from build123d import *

# Parameters (mm, degrees)
SCHIZZO1_R                   = 47
SCHIZZO1_R_2                 = 35
ESTRUSIONE_ESTRUSIONE1_DEPTH = 4
SCHIZZO2_R                   = 2.25
TAGLIO_ESTRUSIONE1_DEPTH     = 4


with BuildPart() as part:
    # Schizzo1 → Estrusione-Estrusione1 (new body)
    with BuildSketch(Plane(origin=(0, 0, 0), x_dir=(1, 0, 0), z_dir=(0, 1, 0))):
        with Locations(Location((0, 0, 0), (0, 0, 270))):
            Circle(SCHIZZO1_R)
        with Locations(Location((0, 0, 0), (0, 0, 270))):
            Circle(SCHIZZO1_R_2, mode=Mode.SUBTRACT)
    extrude(amount=ESTRUSIONE_ESTRUSIONE1_DEPTH)

    # Schizzo2 → Taglio-Estrusione1 (cut)
    with BuildSketch(Plane(origin=(0, 4, 0), x_dir=(1, 0, 0), z_dir=(0, 1, 0))):
        with Locations(Location((0, 41, 0), (0, 0, 270))):
            Circle(SCHIZZO2_R)
        with Locations(Location((41, 0, 0), (0, 0, 270))):
            Circle(SCHIZZO2_R)
        with Locations(Location((0, -41, 0), (0, 0, 270))):
            Circle(SCHIZZO2_R)
        with Locations(Location((-41, 0, 0), (0, 0, 270))):
            Circle(SCHIZZO2_R)
    extrude(amount=-TAGLIO_ESTRUSIONE1_DEPTH, mode=Mode.SUBTRACT)


solid = part.part
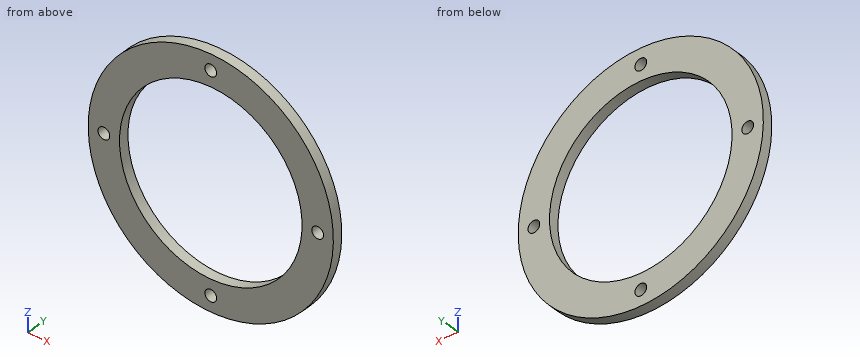
Geometry: final body of the model. Coordinates: model frame, mm. Coordinates: 2 decimals unless noted, no trailing zeros. Loops run counter-clockwise (first coordinate to the right, second up) from the corner with the lowest first, then second, coordinate; pieces in that order, holes last. Notation, with made-up numbers: M 3,41.25 L 44,41.25 A30 ccw 44,65.25 Z; hole C 71.25,37.25 d10. An arc over 180 degrees is marked long. One line per item, written item: value. Start each with the question number.
1) Pin query (flat end, axial travel): P1, Ø7, axis at x = 0, z = -41, coming from the -Y side; P2, Ø1, axis at y = 3.5, z = 29, coming from the +X side; P3, Ø1, axis at y = 3, z = 8, coming from the -X side; P4, Ø4, axis at x = 0, z = 41, coming from the +Y side (1 decimal). Return the tip coordinate at first contact, or that it passes through.
2) Cut plane D-D (z = 1). Return loops of the section in (x, y), then the cut area to 3 significant figures.
3) Cut plane C-C (y = 3.2). Return loops of the section in (x, z), then the cut area to 3 significant figures.
4) Material intervals for L1, parallel to X at y = 1.9, z = 0; L2, parallel to Z at x = -7, y = 2.85; L3, parallel to Z at x = -17, y = 3, sorted ascending. Write a range as from..to.
5) Cut plane B-B (z = 41). Return loops of the section in (x, y).
6) Cut plane A-A (x = -41). Return loops of the section in (y, z), then the cut area to 3 significant figures.
Evaluation:
1. P1: y = 0
1. P2: x = 37.37
1. P3: x = -46.4
1. P4: through
2. outline: M -46.99,0 L -43.02,0 L -43.02,4 L -46.99,4 Z; M -38.98,0 L -34.99,0 L -34.99,4 L -38.98,4 Z; M 34.99,0 L 38.98,0 L 38.98,4 L 34.99,4 Z; M 43.02,0 L 46.99,0 L 46.99,4 L 43.02,4 Z
2. area: 63.8 mm^2
3. outline: C 0,0 d94; hole C -41,0 d4.5; hole C 0,0 d70; hole C 0,-41 d4.5; hole C 0,41 d4.5; hole C 41,0 d4.5
3. area: 3,030 mm^2
4. L1: -47..-43.25, -38.75..-35, 35..38.75, 43.25..47
4. L2: -46.48..-34.29, 34.29..46.48
4. L3: -43.82..-30.59, 30.59..43.82
5. outline: M -22.98,0 L -2.25,0 L -2.25,4 L -22.98,4 Z; M 2.25,0 L 22.98,0 L 22.98,4 L 2.25,4 Z
6. outline: M 0,-22.98 L 4,-22.98 L 4,-2.25 L 0,-2.25 Z; M 0,2.25 L 4,2.25 L 4,22.98 L 0,22.98 Z
6. area: 166 mm^2
